from build123d import *

# Parameters (mm, degrees)
F0_R     = 38.1
F1_DEPTH = 101.6
F4_R     = 3.81


with BuildPart() as f1:
    # F0 (on Top) → F1 (new body)
    with BuildSketch(Plane.XY):
        Circle(F0_R)
        Polygon((-21.997045, 12.7), (0, 25.4), (21.997045, 12.7), (21.997045, -12.7), (0, -25.4), (-21.997045, -12.7), align=None, mode=Mode.SUBTRACT)
    extrude(amount=F1_DEPTH)

    # F2 (on face) → F3 (revolve)
    with BuildSketch(Plane(origin=(21.997045, 0, 0), x_dir=(0, -1, 0), z_dir=(-1, 0, 0))):
        with BuildLine():
            Line((0, 85.725), (0, 79.375))
            ThreePointArc((0, 79.375), (3.175, 82.55), (0, 85.725))
        make_face()
    revolve(axis=Axis((21.997045, 0, 82.55), (0, 0, 1)))

    # F4
    f4_edges = [f1.edges().sort_by_distance(p)[0] for p in [
        (-38.1, 0, 0),
        (-38.1, 0, 101.6),
    ]]
    fillet(f4_edges, radius=F4_R)


solid = f1.part
Can you work these out from the model? Positions are in its coordinate system, mm. A direction names the side the tool comes from. Coordinates: 2 decimals unless noted, no trailing zeros. Loops run counter-clockwise (first coordinate to the right, second up) from the corner with the lowest first, then second, coordinate; pieces in that order, holes last. Notation, with made-up numbers: M -25,5.25 L -12,5.25 A29 cw -12,25.25 Z; hole C -13,-25.5 d10. An arc over 180 degrees is marked long. Return JSON: item names as keys, results as strings. Group by question number.
Item 1: If I drill on L1, parallel to X at y = -16, z = 18.5; L2, parallel to Z at x = -34, y = -6; L3, parallel to Y at x = -17, z = 60.5, over which ranges is the centre line in solid material (lowest first)? Write a range as from..to.
Item 2: Imagine slicing it at B-B (z = 14). Please give me the cut outline in (x, y), and give its area (3 significant figures).
Item 3: Thinking about a two-plate mould opening in X: for faces 3 (the flat face through (22.4, 0.5, 101.6)), 4 (the flat face through (10.84, 19.14, 50.09)), 5 (the flat face through (-11.153, 18.961, 50.089)), 6 (the cylindrical face through (-30.235, -23.183, 50.142)), which applies, released by +X, released by -X, zero draft, split by the parting line, or undercut?
Item 4: I'm going to push flat-ended pins straight in: pin 1 Ø6 at (x, z) = (-7, 91) entering from -Y; pin 2 Ø1 at (x, z) = (14.5, 11.5) entering from +Y; pin 3 Ø1 at (y, z) = (20.5, 74) entering from +X. Where does each tip first touch, or does it pass through?
Item 5: On a 3-axis mill with a long thin cutter (end or side, diameter ignored), from which of +Z, -Z, +X, -X, +Y, -Y can I reach the whole of each face in a straight line? I mean faces 1 (the flat face through (-21.997, 0, 50)), 2 (the flat face through (22.4, 0.5, 0)). Say none if no direction works.
Item 6: Imagine slicing it at A-A (y = 0). Please give me the cut outline in (x, z) (3 decimals).
Verdict:
{
 "1": {"L1": "x = -34.58..-16.28, 16.28..34.58", "L2": "z = 0.01..101.59", "L3": "y = -34.1..-15.59, 15.59..34.1"},
 "2": {"outline": "C 0,0 d76.2; hole M -22,-12.7 L 0,-25.4 L 22,-12.7 L 22,12.7 L 0,25.4 L -22,12.7 Z", "area": "2,880 mm^2"},
 "3": {"face 3": "zero draft", "face 4": "undercut", "face 5": "undercut", "face 6": "split by the parting line"},
 "4": {"pin 1": "stops at y = -37.89", "pin 2": "stops at y = 35.43", "pin 3": "stops at x = 32.43"},
 "5": {"face 1": "+Z, -Z", "face 2": "-Z, +X, -X, +Y, -Y"},
 "6": {"outline": "M -38.1,3.81 A3.81 ccw -34.29,0 L -21.997,0 L -21.997,101.6 L -34.29,101.6 A3.81 ccw -38.1,97.79 Z; M 21.997,0 L 34.29,0 A3.81 ccw 38.1,3.81 L 38.1,97.79 A3.81 ccw 34.29,101.6 L 21.997,101.6 L 21.997,85.725 A3.175 ccw 21.997,79.375 Z"}
}
